Here's how the part is built. I have some questions about the finished solid (model axes, mm). A direction names the side the tool comes from. Give positions to 0.01 mm unless a question says otherwise; leave off trailing zeros. Order: outer loops, then holes, each group sorted by start corner. A loop starts at its lowest first (then second) coordinate and runs counter-clockwise, first axis right, second up. Notation, with made-up numbers: (-17.75, -13) - (23.25, -13) arc R21 cw to (23.25, -9) - close; hole circle Ø7 at (31, 47). An arc over 180 degrees is marked (long way). One line per question, with ' | ' between items.
from build123d import *

# Parameters (mm, degrees)
F2_R      = 19.05
F9_D      = 6.35
F9_DEPTH  = 12.7
F9_TIP    = 1.9077324654
F15_D     = 6.35
F15_DEPTH = 12.7
F15_TIP   = 1.9077324654


with BuildPart() as f3:
    # F3: sweep along a path in F0
    with BuildLine(Plane.XZ) as f3_path:
        Line((-626.3162476942, -437.036204844), (-626.3162476942, 629.763795156))
        Line((-626.3162476942, 629.763795156), (-298.0212476942, 629.763795156))
        Line((-298.0212476942, 629.763795156), (539.3806681667, 217.3478233358))
        Line((539.3806681667, 217.3478233358), (867.6756681667, 217.3478233358))
        Line((867.6756681667, 217.3478233358), (867.6756681667, -849.4521766642))
    # F2 (on plane+point) → F3 (sweep)
    with BuildSketch(Plane.XY.offset(-437.036204844)):
        with Locations((-626.3162476942, 0)):
            Circle(F2_R)
    sweep(path=f3_path.line, transition=Transition.RIGHT)

    # F9 (one way)
    with BuildSketch(Plane.YZ.offset(-607.2662476942)):
        with Locations((0, 572.613795156)):
            Circle(F9_D / 2)
    extrude(amount=-F9_DEPTH, mode=Mode.SUBTRACT)
    with Locations(Plane.YZ.offset(-607.2662476942)):
        with Locations((0, 572.613795156)):
            with Locations((0, 0, -(F9_DEPTH + F9_TIP / 2))):  # 118° drill point
                Cone(0, F9_D / 2, F9_TIP, mode=Mode.SUBTRACT)

    # F15 (one way)
    with BuildSketch(Plane(origin=(848.6256681667, 0, 0), x_dir=(0, -1, 0), z_dir=(-1, 0, 0))):
        with Locations((0, 160.1978233358)):
            Circle(F15_D / 2)
    extrude(amount=-F15_DEPTH, mode=Mode.SUBTRACT)
    with Locations(Plane(origin=(848.6256681667, 0, 0), x_dir=(0, -1, 0), z_dir=(-1, 0, 0))):
        with Locations((0, 160.1978233358)):
            with Locations((0, 0, -(F15_DEPTH + F15_TIP / 2))):  # 118° drill point
                Cone(0, F15_D / 2, F15_TIP, mode=Mode.SUBTRACT)


solid = f3.part
1) I want a section at A-A (z = 119.5). List the corners of the cut face in (x, y) for me, plus the area to 3 significant figures.
Model answer:
outline: circle Ø38.1 at (-626.32, 0); circle Ø38.1 at (867.68, 0) | area: 2,280 mm2
2) I'm going to push flat-ended pins straight in: P1, Ø5, axis at y = -0.5, z = -309, coming from the -X side; P2, Ø12, axis at x = 132, y = -2.5, coming from the +Z side; P3, Ø10, axis at x = -155, y = 9.5, coming from the -Z side; P4, Ø2, axis at x = 336, y = 2, coming from the +Z side. Where does each tip first touch, or does it pass through?
Model answer:
P1: stops at x = -645.37 | P2: stops at z = 442.06 | P3: stops at z = 537.39 | P4: stops at z = 339.13
3) I want a section at B-B (x = 763). List the corners of the cut face in (y, z) for me, plus the area to 3 significant figures.
Model answer:
outline: circle Ø38.1 at (0, 217.35) | area: 1,140 mm2
4) Please list where these lines run through material, in increasing order: L1, parallel to Z at x = 854.25, y = 0; L2, parallel to X at y = 3, z = -135; L3, parallel to X at y = 14.5, z = -91.
Model answer:
L1: z = -849.45 to 157.02, 163.37 to 236.4 | L2: x = -645.13 to -607.5, 848.86 to 886.49 | L3: x = -638.67 to -613.96, 855.32 to 880.03
5) I want a section at C-C (z = -527.5). List the corners of the cut face in (x, y) for me, plus the area to 3 significant figures.
Model answer:
outline: circle Ø38.1 at (867.68, 0) | area: 1,140 mm2
6) On a 3-axis mill with a long thin cutter (end or side, diameter ignored), from which of +Z, -Z, +X, -X, +Y, -Y can I reach the whole of each face in a straight line? I mean faces 1 (the face through (-645.348, 0.838, 113.49)), 2 (the face through (-627, 0, -437.036)), 3 (the face through (-467.013, 0.838, 648.795)). Say none if no direction works.
Model answer:
face 1: -Z | face 2: -Z, -X, +Y, -Y | face 3: none
